Geometry check sheet. Reference: the model listing, model coordinates, mm. A direction names the side the tool comes from. Round coordinates to 2 decimals unless told otherwise and drop trailing zeros. Order: outer loops, then holes, each group sorted by start corner. A loop starts at its lowest first (then second) coordinate and runs counter-clockwise, first axis right, second up.
```python
from build123d import *

# Parameters (mm, degrees)
BOSS_EXTRUDE1_DEPTH = 18.916428128
SKETCH2_R           = 1.25
CUT_EXTRUDE1_DEPTH  = 47.475699972
SKETCH4_R           = 1.55
CUT_EXTRUDE2_DEPTH  = 47.475699972


# Read off the part's stored shape, not the designer's step: Roller coating 12, Roller core 12 coated
with BuildPart() as part:
    # Roller coating 12 outline → Roller coating 12 (revolve)
    with BuildSketch(Plane.YX):
        with BuildLine():
            ThreePointArc((12.7, -17.916428128), (15.217989764, 0), (12.7, 17.916428128))
            Line((12.7, 17.916428128), (8, 17.916428128))
            Line((8, 17.916428128), (8, 17.416428128))
            Line((8, 17.416428128), (12.322080058, 17.416428128))
            ThreePointArc((12.322080058, 17.416428128), (14.717989764, 0), (12.322080058, -17.416428128))
            Line((12.322080058, -17.416428128), (8, -17.416428128))
            Line((8, -17.416428128), (8, -17.916428128))
            Line((8, -17.916428128), (12.7, -17.916428128))
        make_face()
    revolve(axis=Axis((0, 0, 0), (1, 0, 0)))


with BuildPart() as body_2:
    # Roller core 12 coated outline → Roller core 12 coated (revolve)
    with BuildSketch(Plane.YX):
        with BuildLine():
            Line((1.25, 17.416428128), (1.25, -17.416428128))
            Line((1.25, -17.416428128), (12.322080058, -17.416428128))
            ThreePointArc((12.322080058, -17.416428128), (14.717989764, 0), (12.322080058, 17.416428128))
            Line((12.322080058, 17.416428128), (1.25, 17.416428128))
        make_face()
    revolve(axis=Axis((0, 0, 0), (1, 0, 0)))


with BuildPart() as part_1:
    add(part.part)

    # Combine1: union body 2
    add(body_2.part)


with BuildPart() as body_2_2:
    # Sketch1 → Revolve1 (revolve)
    with BuildSketch(Plane.XY, mode=Mode.PRIVATE) as revolve1_sk:
        with BuildLine():
            Line((0, 0), (0, 15.217989764))
            Line((0, 15.217989764), (0, 16.017989764))
            ThreePointArc((0, 16.017989764), (-9.046251562, 15.385414232), (-17.916428128, 13.5))
            Line((-17.916428128, 13.5), (-18.916428128, 13.5))
            Line((-18.916428128, 13.5), (-18.916428128, 0))
            Line((-18.916428128, 0), (0, 0))
        make_face()
    revolve(revolve1_sk.sketch.rotate(Axis((-18.916428128, 0, 0), (1, 0, 0)), 270), axis=Axis((-18.916428128, 0, 0), (1, 0, 0)))

    # Sketch3 → Boss-Extrude1 (add)
    with BuildSketch(Plane(origin=(-18.916428128, 0, 0), x_dir=(0, 0, -1), z_dir=(1, 0, 0))):
        with BuildLine():
            Line((-3.5, 26.517989764), (-3.5, 13.03840481))
            ThreePointArc((-3.5, 13.03840481), (-9.545941546, 9.545941546), (-13.03840481, 3.5))
            Line((-13.03840481, 3.5), (-26.517989764, 3.5))
            ThreePointArc((-26.517989764, 3.5), (-30.017989764, 0), (-26.517989764, -3.5))
            Line((-26.517989764, -3.5), (-13.03840481, -3.5))
            ThreePointArc((-13.03840481, -3.5), (-9.545941546, -9.545941546), (-3.5, -13.03840481))
            Line((-3.5, -13.03840481), (-3.5, -26.517989764))
            ThreePointArc((-3.5, -26.517989764), (0, -30.017989764), (3.5, -26.517989764))
            Line((3.5, -26.517989764), (3.5, -13.03840481))
            ThreePointArc((3.5, -13.03840481), (9.545941546, -9.545941546), (13.03840481, -3.5))
            Line((13.03840481, -3.5), (26.517989764, -3.5))
            ThreePointArc((26.517989764, -3.5), (30.017989764, 0), (26.517989764, 3.5))
            Line((26.517989764, 3.5), (13.03840481, 3.5))
            ThreePointArc((13.03840481, 3.5), (9.545941546, 9.545941546), (3.5, 13.03840481))
            Line((3.5, 13.03840481), (3.5, 26.517989764))
            ThreePointArc((3.5, 26.517989764), (0, 30.017989764), (-3.5, 26.517989764))
        make_face()
    extrude(amount=BOSS_EXTRUDE1_DEPTH)

    # Combine2: cut part
    add(part_1.part, mode=Mode.SUBTRACT)

    # Sketch2 → Cut-Extrude1 (cut, through all)
    with BuildSketch(Plane(origin=(0, 0, 0), x_dir=(0, 0, -1), z_dir=(1, 0, 0))):
        Circle(SKETCH2_R)
    extrude(amount=-CUT_EXTRUDE1_DEPTH, mode=Mode.SUBTRACT)

    # Sketch4 → Cut-Extrude2 (cut, through all)
    with BuildSketch(Plane(origin=(0, 0, 0), x_dir=(0, 0, -1), z_dir=(1, 0, 0))):
        with Locations((0, -26.517989764)):
            Circle(SKETCH4_R)
        with Locations((-26.517989764, 0)):
            Circle(SKETCH4_R)
        with Locations((0, 26.517989764)):
            Circle(SKETCH4_R)
        with Locations((26.517989764, 0)):
            Circle(SKETCH4_R)
    extrude(amount=-CUT_EXTRUDE2_DEPTH, mode=Mode.SUBTRACT)


solid = body_2_2.part
```
(1) Sectioned sample at A-A, the plane y = 0. Give the number of separate pieces and of enclosed holes in the cut face, and give its area (3 significant figures).
Returned:
separate pieces: 4
enclosed holes: 0
area: 507 mm2
(2) Material ranges on line 1 (Y direction, x = -18.45, z = 0); line 2 (Y direction, x = -13.25, z = 26.5); line 3 (Z direction, x = -16.5, y = -19.5), recorded low to high.
Returned:
line 1: y = -30.02 to -28.07, -24.97 to -1.25, 1.25 to 24.97, 28.07 to 30.02
line 2: y = -3.5 to -1.55, 1.55 to 3.5
line 3: z = -3.5 to 3.5
(3) Set-up check for faces 1 (the cylindrical face through (-18.423, -9.476, 9.616)), 2 (the cylindrical face through (-18.423, -9.616, -9.476)), 3 (the cylindrical face through (-9.591, -0.077, -30.017)), 4 (the cylindrical face through (-18.423, 9.476, -9.616)): record each of +Z, -Z, +X, -X, +Y, -Y from which the full face is reachable in a straight line by a thin tool's end or side.
Returned:
face 1: +Z, -X, -Y
face 2: -Z, -X, -Y
face 3: -Z, +X, -X
face 4: -Z, -X, +Y
(4) Depth check by flat-ended pin: P1, Ø4, axis at x = -9, y = -19, coming from the -Z side; P2, Ø11, axis at x = -10, z = -17, coming from the +Y side; P3, Ø4, axis at x = -12, y = 10, coming from the -Z side; P4, Ø12, axis at y = 3, z = 19, coming from the +X side. Enter the tip coordinate at first touch or a pass-through.
Returned:
P1: stops at z = -3.5
P2: stops at y = 10.13
P3: stops at z = -12.64
P4: stops at x = 0
(5) Sectioned sample at C-C, the plane y = 22. Record the cut outline in (x, z).
Returned:
outline: (-18.92, -3.5) - (0, -3.5) - (0, 3.5) - (-18.92, 3.5) - close
(6) Draft check along Y on faces 5 (the flat face through (-17.416, 0, -2)), 6 (the cylindrical face through (-9.591, 30.017, -0.077)), 7 (the cylindrical face through (-9.591, 0.077, 30.017)). Enter one of: released by +Y, released by -Y, zero draft, split by the parting line, or undercut.
Returned:
face 5: undercut
face 6: released by +Y
face 7: split by the parting line
